from build123d import *

# Parameters (mm, degrees)
SKETCH1_W           = 40
SKETCH1_H           = 3
BOSS_EXTRUDE1_DEPTH = 3
SKETCH3_R           = 1.5
SKETCH3_W           = 12
SKETCH3_H           = 20
SKETCH3_W_2         = 60
CUT_EXTRUDE2_DEPTH  = 10


with BuildPart() as part:
    # Sketch1 → Boss-Extrude1 (new body)
    with BuildSketch(Plane(origin=(0, 0, 0), x_dir=(1, 0, 0), z_dir=(0, 1, 0))):
        Polygon((20, 37.5), (20, 12.5), (0, 12.5), (0, 0), (10, 0), (10, -40), (70, -40), (70, 0), (80, 0), (80, 12.5), (60, 12.5), (60, 37.5), (80, 37.5), (80, 50), (70, 50), (70, 90), (10, 90), (10, 50), (0, 50), (0, 37.5), align=None)
        with Locations((40, -4.5)):
            Rectangle(SKETCH1_W, SKETCH1_H, mode=Mode.SUBTRACT)
        with Locations((40, 54.5)):
            Rectangle(SKETCH1_W, SKETCH1_H, mode=Mode.SUBTRACT)
    extrude(amount=BOSS_EXTRUDE1_DEPTH)

    # Sketch3 → Cut-Extrude2 (cut)
    with BuildSketch(Plane(origin=(0, 0, 0), x_dir=(1, 0, 0), z_dir=(0, 1, 0))):
        with Locations(Location((16, -32.25, 0), (0, 0, 270))):
            Circle(SKETCH3_R)
        with Locations(Location((16, -14.75, 0), (0, 0, 270))):
            Circle(SKETCH3_R)
        with Locations((40, -30)):
            Rectangle(SKETCH3_W, SKETCH3_H)
        with Locations((40, 80)):
            Rectangle(SKETCH3_W_2, SKETCH3_H)
    extrude(amount=CUT_EXTRUDE2_DEPTH, mode=Mode.SUBTRACT)


solid = part.part
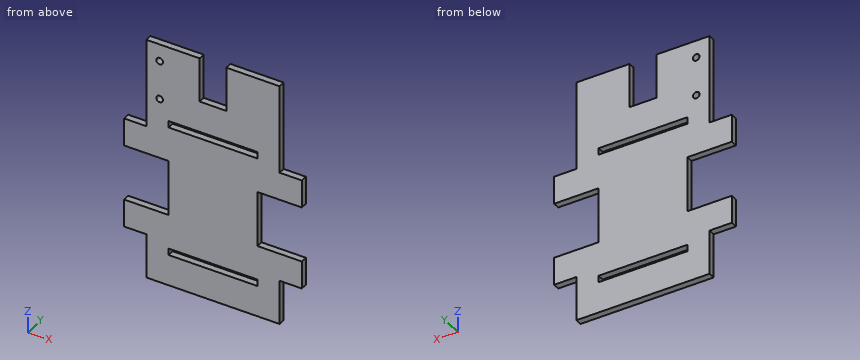
The model under review builds one solid part; all positions refer to its coordinate system, in mm. Give positions to 0.01 mm unless a question says otherwise; leave off trailing zeros. Write each loop counter-clockwise with the first axis right and the second up, starting at its lowest first coordinate (ties: lowest second). Pieces come first, ordered by that corner, then holes. Notation, with made-up numbers: M -21,78 L 32,78 A16 cw 32,84 Z; hole C 84.5,33 d3. An arc over 180 degrees is marked long. One line per question, with ' | ' between items. Start each with the question number.
Item 1: We need section C-C on x = 73.5. Write out the cut boundary in (y, z).
Item 2: We need section D-D on z = 14.75. Write out the cut boundary in (x, y).
Item 3: We need section A-A on z = 32.25. Write out the cut boundary in (x, y), plus the area to 3 significant figures.
Item 4: We need section B-B on x = 44.5. Write out the cut boundary in (y, z).
Item 5: For pin 1 (0.9 mm diameter, centred on y = 1.5, z = 5, fed in from +X); pin 2 (0.9 mm diameter, centred on y = 2, z = -21.5, fed in from +X); pin 3 (1.5 mm diameter, centred on y = 1, z = -29, fed in from -X), all flat-tipped, find the tip position at first contact; note any pin that passes through.
Item 6: Wall thickness on line 1 (Z direction, x = 16, y = 1.45); line 2 (Z direction, x = 54.5, y = 2.25); line 3 (Z direction, x = 44.5, y = 2.2): over which ranges is each line inside the solid? List them lowest first. Write a range as from..to.
Results found:
1) outline: M 0,-50 L 3,-50 L 3,-37.5 L 0,-37.5 Z; M 0,-12.5 L 3,-12.5 L 3,0 L 0,0 Z
2) outline: M 10,0 L 14.5,0 L 14.5,3 L 10,3 Z; M 17.5,0 L 70,0 L 70,3 L 17.5,3 Z
3) outline: M 10,0 L 14.5,0 L 14.5,3 L 10,3 Z; M 17.5,0 L 34,0 L 34,3 L 17.5,3 Z; M 46,0 L 70,0 L 70,3 L 46,3 Z | area: 135 mm2
4) outline: M 0,-70 L 3,-70 L 3,-56 L 0,-56 Z; M 0,-53 L 3,-53 L 3,3 L 0,3 Z; M 0,6 L 3,6 L 3,20 L 0,20 Z
5) pin 1: stops at x = 70 | pin 2: stops at x = 60 | pin 3: stops at x = 20
6) line 1: z = -70..-37.5, -12.5..13.25, 16.25..30.75, 33.75..40 | line 2: z = -70..-56, -53..3, 6..40 | line 3: z = -70..-56, -53..3, 6..20
